Check sheet for the modelled part. Datum: model origin and axes. Units: mm. A direction names the side the tool comes from. Give positions to 0.01 mm unless a question says otherwise; leave off trailing zeros. Write each loop counter-clockwise with the first axis right and the second up, starting at its lowest first coordinate (ties: lowest second). Pieces come first, ordered by that corner, then holes. Notation, with made-up numbers: M -33,21.5 L 9,21.5 A12 cw 9,32.5 Z; hole C 73.25,53.25 d1. An arc over 180 degrees is marked long. Write item = value, one per line. Start each with the question number.
1) Gauge pin test, flat ends, axial feed: pin 1 (3.5 mm diameter, centred on x = -1.5, z = -5.5, fed in from +Y) (3 decimals); pin 2 (2.5 mm diameter, centred on x = 0, y = -10, fed in from +Z); pin 3 (2 mm diameter, centred on x = -4, z = -1.5, fed in from -Y) (3 decimals); pin 4 (1.5 mm diameter, centred on x = 0.5, y = -1.5, fed in from -Z). Record the tip position at first contact, or that the pin passes through.
2) Set-up check for faces 4 (the face through (-1, -4, 2)), 5 (the face through (6.988, -9, -12)), 6 (the face through (0, 0, 0)), 7 (the face through (1, -7.735, -5)): record each of +Z, -Z, +X, -X, +Y, -Y from which the full face is reachable in a straight line by a thin tool's end or side.
3) Sectioned sample at C-C, the plane y = -3. Record the cut outline in (x, z).
4) Sectioned sample at B-B, the plane x = 0.75. Record the cut outline in (y, z) (3 decimals), then the cut area to 3 significant figures.
5) Sectioned sample at D-D, the plane y = 0.25. Record the cut outline in (x, z).
6) Draft check along X on faces 1 (the face through (-5.976, -6, -5)), 2 (the face through (0.26, -4.08, 0.89)), 3 (the face through (0, 1.765, 1)). Enter one of: pulls with the +X half, pulls with the -X half, needs draft (parallel to the pull), parting line crosses it, or undercut.
7) Scan lines: L1, parallel to Z at x = -2, y = -10.5; L2, parallel to Y at x = 0.5, z = -8 (3 decimals); L3, parallel to Z at x = 4.25, y = -3. Record each from-to range of solid material in increasing order.
8) Sectioned sample at A-A, the plane x = -4.75. Record the cut outline in (y, z) (3 decimals), then the cut area to 3 significant figures.
Autodesk Inventor part; units mm, degrees
ref_plane "YZ Plane" through (0, 0, 0) normal (1, 0, 0) x (0, 1, 0)
ref_plane "XZ Plane" through (0, 0, 0) normal (0, 1, 0) x (-1, 0, 0)
ref_plane "XY Plane" through (0, 0, 0) normal (0, 0, 1) x (1, 0, 0)
sketch "Sketch1" plane through (0, 0, 0) normal (0, 0, 1) x (1, 0, 0)
  line L0 (-5.976, 1.765) -> (7.024, 1.765)
  line L1 (7.024, 1.765) -> (7.024, -7.735)
  line L2 (7.024, -7.735) -> (-5.976, -7.735)
  line L3 (-5.976, -7.735) -> (-5.976, 1.765)
  line L4 (-5.976, -7.735) -> (7.024, -7.735)
  line L5 (7.024, -7.735) -> (7.024, -5.235)
  line L6 (7.024, -5.235) -> (-5.976, -5.235)
  line L7 (-5.976, -5.235) -> (-5.976, -7.735)
  circle A0 centre (0.524, -2.0964) radius 2
  point P0 (0, 0)
  dimension "d0" = 9.5
  dimension "d1" = 13
  dimension "d2" = 2.5
  dimension "d3" = 4
  dimension "d4" = 6.5
  dimension "d5" = 3.8614
extrude "Extrusion1" add sketch "Sketch1" along normal blind 2
extrude "Extrusion2" add sketch "Sketch1" against normal blind 11.2 contours L6 L1 L2 L3
sketch "Sketch2" plane through (0, 0, -11.2) normal (0, 0, -1) x (-1, 0, 0)
  line L0 (-6.988, -5.235) -> (5.976, -5.235)
  line L1 (5.976, -5.235) -> (5.976, -13.235)
  line L2 (5.976, -13.235) -> (-6.988, -13.235)
  line L3 (-6.988, -13.235) -> (-6.988, -5.235)
  line L4 (5.976, -7.735) -> (5.976, -5.235)
  line L5 (5.976, -5.235) -> (-7.024, -5.235)
  point P0 (0, 0)
  dimension "d10" = 0
  dimension "d11" = 8
  dimension "d12" = 0
extrude "Extrusion3" add sketch "Sketch2" along normal blind 2
fillet "Fillet1" radius 2 1 edges at (0.524, -5.235, 0)
properties part number "ethernet bracket support"
Data:
q1.pin_1 = -5.235
q1.pin_2 = -11.2
q1.pin_3 = -7.735
q1.pin_4 = through
q2.face_4 = +Z, +X, -X, +Y, -Y
q2.face_5 = -Z, +X, +Y, -Y
q2.face_6 = -Z, +X, -X, +Y
q2.face_7 = +Z, +X, -X, -Y
q3.outline = M -5.98,0 L -1.26,0 L -1.26,2 L -5.98,2 Z; M 2.31,0 L 7.02,0 L 7.02,2 L 2.31,2 Z
q4.outline = M -13.235,-13.2 L -5.235,-13.2 L -5.235,-2 A2 cw -4.084,-0.189 L -4.084,2 L -7.735,2 L -7.735,-11.2 L -13.235,-11.2 Z; M -0.109,0 L 1.765,0 L 1.765,2 L -0.109,2 Z
q4.area = 55.9 mm2
q5.outline = M -5.98,0 L 7.02,0 L 7.02,2 L -5.98,2 Z
q6.face_1 = pulls with the -X half
q6.face_2 = undercut
q6.face_3 = needs draft
q7.L1 = -13.2 to -11.2
q7.L2 = -7.735 to -5.235
q7.L3 = 0 to 2
q8.outline = M -13.235,-13.2 L -5.235,-13.2 L -5.235,-2 A2 cw -3.235,0 L 1.765,0 L 1.765,2 L -7.735,2 L -7.735,-11.2 L -13.235,-11.2 Z
q8.area = 63.9 mm2
